Autodesk Inventor part; units mm, degrees
ref_plane "YZ Plane" through (0, 0, 0) normal (1, 0, 0) x (0, 1, 0)
ref_plane "XZ Plane" through (0, 0, 0) normal (0, 1, 0) x (-1, 0, 0)
ref_plane "XY Plane" through (0, 0, 0) normal (0, 0, 1) x (1, 0, 0)
sketch "Sketch1" plane through (0, 0, 0) normal (1, 0, 0) x (0, 1, 0)
  line L0 (0, 0) -> (0, 23.5)
  line L1 (0, 23.5) -> (6, 23.5)
  line L2 (6, 23.5) -> (6, -23.5)
  line L3 (6, -23.5) -> (0, -23.5)
  line L4 (0, -23.5) -> (0, 0)
  line L5 (6, 23.5) -> (6, 21.5)
  line L6 (6, 21.5) -> (4, 21.5)
  circle A0 centre (4, 21.5) radius 2
  line L7 (6, -23.5) -> (6, -21.5)
  line L8 (6, -21.5) -> (4, -21.5)
  circle A1 centre (4, -21.5) radius 2
  line L9 (6, -23.5) -> (6, -16.5)
  line L10 (6, -16.5) -> (3, -16.5)
  line L11 (6, 23.5) -> (6, 16.5)
  line L12 (6, 16.5) -> (3, 16.5)
  circle A2 centre (3, 16.5) radius 2
  circle A3 centre (3, -16.5) radius 2
  point P0 (4, 23.5)
  point P1 (4, -23.5)
  dimension "d0" = 23.5
  dimension "d1" = 6
  dimension "d2" = 47
  dimension "d3" = 6
  dimension "d4" = 2
  dimension "d5" = 2
  dimension "d6" = 4
  dimension "d7" = 2
  dimension "d8" = 2
  dimension "d9" = 4
  dimension "d10" = 7
  dimension "d11" = 3
  dimension "d12" = 7
  dimension "d13" = 3
  dimension "d14" = 4
  dimension "d15" = 4
extrude "Extrusion1" add sketch "Sketch1" along normal blind 7.2555 contours L0 L1 A0 L2 A1 L3 L4 | A0 | A1
sketch "Sketch2" plane through (0, 6, 21.5) normal (0, 1, 0) x (1, 0, 0)
  line L0 (7.2555, -2) -> (7.2555, 0)
  line L1 (0, 0) -> (7.2555, 0)
  line L2 (7.2555, 0) -> (0, 0)
  line L3 (0, 0) -> (0, 43)
  line L4 (0, -2) -> (0, 45)
  line L5 (0, 43) -> (7.2555, 43)
  line L6 (7.2555, 43) -> (7.2555, 0)
  point P0 (0, 21.5)
  dimension "d18" = 7.2555
  dimension "d19" = 43
  dimension "d20" = 7.2555
extrude "Extrusion2" add sketch "Sketch2" along normal blind 25
sketch "Sketch3" plane through (0, 0, 0) normal (-1, 0, 0) x (0, 0, 1)
  arc A0 (23.5, 4) -> (21.5, 6) centre (21.5, 4) ccw
  line L0 (21.5, 6) -> (21.5, 8)
  line L1 (21.5, 6) -> (21.5, 31)
  circle A1 centre (21.5, 8) radius 2
  line L2 (19.5, 8) -> (19.5, 31)
  line L3 (21.5, 31) -> (-21.5, 31)
  line L4 (19.5, 31) -> (21.5, 31)
  line L5 (21.5, 31) -> (21.5, 10)
  line L6 (-21.5, 6) -> (-21.5, 31)
  line L7 (-21.5, 6) -> (-21.5, 8)
  circle A2 centre (-21.5, 8) radius 2
  line L8 (-19.5, 8) -> (-19.5, 31)
  line L9 (-19.5, 31) -> (-21.5, 31)
  line L10 (-21.5, 31) -> (-21.5, 10)
  point P0 (0, 0)
  dimension "d23" = 2
  dimension "d24" = 4
  dimension "d25" = 23
  dimension "d26" = 2
  dimension "d27" = 4
  dimension "d28" = 23
extrude "Extrusion3" cut sketch "Sketch3" against normal blind 7.2555 contours A1 L1 L0 | L8 A2 L6 L3 | L2 L3 L1 A1 | A2 L6 picked at (20.5631, 8.9369) picked at (-20.5631, 7.0631)
sketch "Sketch4" plane through (7.2555, 0, 0) normal (1, 0, 0) x (0, 0, -1)
  line L0 (-19.5, 31) -> (19.5, 31)
  line L1 (-19.5, 31) -> (-19.5, 26)
  line L2 (-19.5, 8) -> (-19.5, 31)
  line L3 (-19.5, 26) -> (19.5, 26)
  line L4 (19.5, 26) -> (19.5, 31)
  line L5 (-19.5, 31) -> (19.5, 31)
  point P0 (0, 0)
  dimension "d31" = 5
  dimension "d32" = 39
extrude "Extrusion4" add sketch "Sketch4" along normal blind 27.422
sketch "Sketch5" plane through (0, 8, 19.5) normal (0, 0, 1) x (1, 0, 0)
  line L0 (0, 0) -> (0, 23)
  line L1 (0, 23) -> (0, 21)
  line L2 (0, 21) -> (2, 21)
  circle A0 centre (2, 21) radius 2
  line L3 (0, 23) -> (2, 23)
  line L4 (0, 23) -> (34.6775, 23)
  line L5 (7.2555, 18) -> (34.6775, 18)
  line L6 (7.2555, 18) -> (7.2555, 16)
  line L7 (7.2555, 16) -> (9.2555, 16)
  circle A1 centre (9.2555, 16) radius 2
  line L8 (7.2555, 18) -> (9.2555, 18)
  point P0 (0, -8)
  point P1 (7.2555, 16)
  dimension "d37" = 4
  dimension "d40" = 4
  dimension "d35" = 2
  dimension "d36" = 2
  dimension "d38" = 2
  dimension "d39" = 2
extrude "Extrusion5" cut sketch "Sketch5" against normal blind 39 contours L0 L3 A0 | L5 A1 L6
sketch "Sketch6" plane through (0, 8, 19.5) normal (0, 0, 1) x (1, 0, 0)
  line L0 (7.2555, 18) -> (7.2555, 0)
  line L1 (7.2555, 18) -> (7.2555, 16)
  line L2 (7.2555, 16) -> (9.2555, 16)
  circle A0 centre (9.2555, 16) radius 2
  line L3 (7.2555, 18) -> (34.6775, 18)
  line L4 (7.2555, 18) -> (9.2555, 18)
  point P0 (0, -8)
  point P1 (7.2555, 16)
  dimension "d45" = 4
  dimension "d43" = 2
  dimension "d44" = 2
extrude "Extrusion6" add sketch "Sketch6" against normal blind 39 contours L3 A0 L0
sketch "Sketch7" plane through (34.6775, 0, 0) normal (1, 0, 0) x (0, 0, -1)
  line L0 (-19.5, 31) -> (-19.5, 26)
  line L1 (19.5, 26) -> (19.5, 31)
  line L2 (-19.5, 31) -> (19.5, 31)
  line L3 (19.5, 31) -> (19.5, 26)
  line L4 (19.5, 26) -> (-19.5, 26)
  line L5 (-19.5, 26) -> (-19.5, 31)
  point P0 (0, 0)
extrude "Extrusion7" add sketch "Sketch7" along normal blind 5
sketch "Sketch8" plane through (0, 8, 19.5) normal (0, 0, 1) x (1, 0, 0)
  line L0 (39.6775, 23) -> (2, 23)
  line L1 (39.6775, 23) -> (37.6775, 23)
  line L2 (37.6775, 23) -> (37.6775, 21)
  circle A0 centre (37.6775, 21) radius 2
  line L3 (39.6775, 23) -> (39.6775, 21)
  point P0 (0, -8)
  dimension "d52" = 4
  dimension "d50" = 2
  dimension "d51" = 2
extrude "Extrusion8" cut sketch "Sketch8" against normal blind 39 contours L3 A0 L0
sketch "Sketch9" plane through (9.2555, 26, -19.5) normal (0, -1, 0) x (1, 0, 0)
  line L0 (30.422, 39) -> (30.422, 0)
  line L1 (30.422, 39) -> (25.422, 39)
  line L2 (0, 39) -> (30.422, 39)
  line L3 (25.422, 39) -> (25.422, 0)
  line L4 (25.422, 0) -> (30.422, 0)
  line L5 (30.422, 0) -> (30.422, 39)
  point P0 (-9.2555, 19.5)
  dimension "d55" = 5
  dimension "d56" = 39
extrude "Extrusion9" add sketch "Sketch9" along normal blind 34
sketch "Sketch10" plane through (39.6775, 0, 0) normal (1, 0, 0) x (0, 0, -1)
  line L0 (-19.5, 31) -> (-19.5, 29)
  line L1 (-19.5, 29) -> (-19.5, 26)
  line L2 (-19.5, 29) -> (-19.5, -8)
  line L3 (-19.5, 26) -> (19.5, 26)
  line L4 (19.5, 26) -> (19.5, 29)
  line L5 (19.5, 29) -> (-19.5, 29)
  line L6 (-19.5, 26) -> (-9.933, 26)
  line L7 (-9.933, 26) -> (-9.933, 13.756)
  line L8 (-9.933, 13.756) -> (-7.383, 13.756)
  line L9 (-7.383, 13.756) -> (-7.383, 11.556)
  line L10 (-7.383, 11.556) -> (-7.383, 9.356)
  line L11 (-7.383, 9.356) -> (-12.483, 9.356)
  line L12 (-12.483, 9.356) -> (-12.483, 11.556)
  line L13 (-12.483, 11.556) -> (-12.483, 13.756)
  line L14 (-12.483, 13.756) -> (-9.933, 13.756)
  circle A0 centre (-7.383, 11.556) radius 2.2
  circle A1 centre (-12.483, 11.556) radius 2.2
  line L15 (19.5, 26) -> (21.044, 26)
  line L16 (21.044, 26) -> (21.044, 11.5)
  circle A2 centre (21.044, 11.5) radius 2.5
  point P0 (0, 0)
  dimension "d59" = 3
  dimension "d60" = 39
  dimension "d61" = 9.567
  dimension "d62" = 12.244
  dimension "d63" = 2.55
  dimension "d64" = 2.2
  dimension "d65" = 2.2
  dimension "d66" = 5.1
  dimension "d67" = 2.2
  dimension "d68" = 2.2
  dimension "d69" = 4.4
  dimension "d70" = 4.4
  dimension "d71" = 1.544
  dimension "d72" = 14.5
  dimension "d73" = 5
extrude "Extrusion10" cut sketch "Sketch10" against normal blind 5 contours A2 | L8 A0 L11 A1 L14 | A0 L10 L9 | L9 L10 A0 | A1 L12 L13 | L13 L12 A1
sketch "Sketch11" plane through (34.6775, 26, -19.5) normal (-1, 0, 0) x (0, 0, 1)
  line L0 (39, -34) -> (0, -34)
  line L1 (39, -34) -> (39, -26)
  line L2 (39, 3) -> (39, -34)
  line L3 (39, -26) -> (0, -26)
  line L4 (0, -26) -> (0, -34)
  line L5 (0, -34) -> (39, -34)
  point P0 (19.5, -26)
  dimension "d76" = 8
  dimension "d77" = 39
extrude "Extrusion11" add sketch "Sketch11" along normal blind 6.58
sketch "Sketch12" plane through (0, 8, 19.5) normal (0, 0, 1) x (1, 0, 0)
  line L0 (39.6775, 21) -> (39.6775, -16)
  line L1 (39.6775, -16) -> (37.6775, -16)
  line L2 (39.6775, -16) -> (28.0975, -16)
  line L3 (37.6775, -16) -> (37.6775, -14)
  circle A0 centre (37.6775, -14) radius 2
  line L4 (39.6775, -16) -> (39.6775, -14)
  point P0 (0, -8)
  point P1 (37.6775, -16)
  dimension "d82" = 4
  dimension "d80" = 2
  dimension "d81" = 2
extrude "Extrusion12" cut sketch "Sketch12" against normal blind 39 contours L0 L1 A0
properties part number "camera_lock"
Part model, mm, in its own coordinate system. A direction names the side the tool comes from. Coordinates: 2 decimals unless noted, no trailing zeros. Write each loop counter-clockwise with the first axis right and the second up, starting at its lowest first coordinate (ties: lowest second). Pieces come first, ordered by that corner, then holes. Notation, with made-up numbers: (58, 86.25) - (72, 86.25) arc R7 ccw to (72, 99.25) - close; hole circle Ø10 at (47.5, 58.5). An arc over 180 degrees is marked (long way). Put each result on its own line as item: value.
1. Band-saw the part on D-D (y = 3). Write the cut outline in (x, z), then the cut area to 3 significant figures.
Final values:
outline: (0, -23.5) - (7.26, -23.5) - (7.26, -18.5) - (0, -18.5) - close; (0, -14.5) - (7.26, -14.5) - (7.26, 14.5) - (0, 14.5) - close; (0, 18.5) - (7.26, 18.5) - (7.26, 23.5) - (0, 23.5) - close; (34.68, -19.5) - (39.68, -19.5) - (39.68, 19.5) - (34.68, 19.5) - close
area: 478 mm²
2. 3-axis set-ups, long thin cutter, end or side, ignore diameter. For faces 5 (the flat face through (22, 26, 0)), 6 (the cylindrical face through (37.213, 11.532, -18.544)), 7 (the flat face through (7.256, 12, 0)): which of +Z, -Z, +X, -X, +Y, -Y reach the whole face in a straight line?
Final values:
face 5: +Z, -Z
face 6: -Z, +X
face 7: +Z, -Z, -Y
3. Band-saw the part on B-B (y = 14.5). Write the cut outline in (x, z).
Final values:
outline: (0, -19.5) - (7.26, -19.5) - (7.26, 19.5) - (0, 19.5) - close; (34.68, -19.5) - (39.68, -19.5) - (39.68, 19.5) - (34.68, 19.5) - close
4. Band-saw the part on A-A (x = 32). Write the cut outline in (y, z).
Final values:
outline: (-8, -19.5) - (0, -19.5) - (0, 19.5) - (-8, 19.5) - close; (26, -19.5) - (31, -19.5) - (31, 19.5) - (26, 19.5) - close
5. Two-plate mould, pull along Y, no slides. Class faces 1 (the cylindrical face through (39.076, -7.43, 0.273)), 2 (the cylindrical face through (0.6, 30.43, 0.27)), 3 (the flat face through (34.678, 13, 0)), 4 (the flat face through (35, -1, -19.5)): +Y half, -Y half, draft (parallel to the pull), parting line (faces both ways), or undercut.
Final values:
face 1: -Y half
face 2: +Y half
face 3: undercut
face 4: draft
6. Flat gauge pins, fed straight in: pin 1 Ø12 at (x, z) = (4, 3.5) entering from -Y; pin 2 Ø12.5 at (x, y) = (36, -1.5) entering from -Z; pin 3 Ø2.5 at (y, z) = (-5.5, 9) entering from -X; pin 4 Ø8 at (x, y) = (30, 9) entering from +Z. Where does each tip first touch, or does it go through?
Final values:
pin 1: stops at y = 0
pin 2: stops at z = -19.5
pin 3: stops at x = 28.1
pin 4: passes through
7. Band-saw the part on C-C (z = 16.5). Write the cut outline in (x, y), then the cut area to 3 significant figures.
Final values:
outline: (0, 0) - (7.26, 0) - (7.26, 1) - (0, 1) - close; (0, 5) - (7.26, 5) - (7.26, 24) arc R2 cw to (9.26, 26) - (34.68, 26) - (34.68, 0) - (28.1, 0) - (28.1, -8) - (37.68, -8) arc R2 ccw to (39.68, -6) - (39.68, 29) arc R2 ccw to (37.68, 31) - (2, 31) arc R2 ccw to (0, 29) - close
area: 579 mm²
8. Probe line 1 along Z through (x, y) = (3, 3); line 2 along X through (y, z) = (6, 13.5); line 3 along Z through (x, y) = (5.5, 12.5). List the from-to ranges inside material, lowest first. Write a range as [from, to].
Final values:
line 1: z = [-23.5, -18.5], [-14.5, 14.5], [18.5, 23.5]
line 2: x = [0, 7.26], [34.68, 39.68]
line 3: z = [-19.5, 19.5]
